```python
from build123d import *

# Parameters (mm, degrees)
SKETCH1_W           = 88
SKETCH1_H           = 92
BOSS_EXTRUDE1_DEPTH = 2
FILLET1_R           = 4
SKETCH3_W           = 28
SKETCH3_H           = 2
SKETCH3_W_2         = 9
BOSS_EXTRUDE3_DEPTH = 3
SKETCH4_W           = 2
SKETCH4_H           = 5
BOSS_EXTRUDE4_DEPTH = 6
FILLET2_R           = 2
BOSS_EXTRUDE5_DEPTH = 2
FILLET4_R           = 0.5


with BuildPart() as part:
    # Sketch1 → Boss-Extrude1 (new body)
    with BuildSketch(Plane.XY):
        with Locations((-29.854657196, 17.8829867)):
            Rectangle(SKETCH1_W, SKETCH1_H)
    extrude(amount=BOSS_EXTRUDE1_DEPTH)

    # Fillet1
    fillet1_edges = [part.edges().sort_by_distance(p)[0] for p in [
        (-73.854657196, 63.8829867, 1),
        (14.145342804, 63.8829867, 1),
    ]]
    fillet(fillet1_edges, radius=FILLET1_R)

    # Sketch3 → Boss-Extrude3 (add)
    with BuildSketch(Plane(origin=(0, 0, 0), x_dir=(-1, 0, 0), z_dir=(0, 0, -1))):
        with Locations((56.354657196, 62.8829867)):
            Rectangle(SKETCH3_W, SKETCH3_H)
        with Locations((29.854657196, 62.8829867)):
            Rectangle(SKETCH3_W_2, SKETCH3_H)
        with Locations((3.354657196, 62.8829867)):
            Rectangle(SKETCH3_W, SKETCH3_H)
    extrude(amount=BOSS_EXTRUDE3_DEPTH)

    # Sketch4 → Boss-Extrude4 (add)
    with BuildSketch(Plane(origin=(0, 0, 0), x_dir=(-1, 0, 0), z_dir=(0, 0, -1))):
        with Locations((-13.145342804, 21.3829867)):
            Rectangle(SKETCH4_W, SKETCH4_H)
    extrude(amount=BOSS_EXTRUDE4_DEPTH)

    # Fillet2
    fillet2_edges = [part.edges().sort_by_distance(p)[0] for p in [
        (14.145342804, -28.1170133, 1),
        (-73.854657196, -28.1170133, 1),
    ]]
    fillet(fillet2_edges, radius=FILLET2_R)

    # Sketch5 → Boss-Extrude5 (add)
    with BuildSketch(Plane(origin=(0, 0, 0), x_dir=(-1, 0, 0), z_dir=(0, 0, -1))):
        Polygon((71.854657196, -26.1170133), (68.854657196, -26.1170133), (-12.145342804, -26.1170133), (-12.145342804, -23.1170133), (-12.145342804, 54.889958553), (-9.145342804, 54.889958553), (-9.145342804, -23.1170133), (68.854657196, -23.1170133), (68.854657196, 54.749214955), (71.854657196, 54.749214955), align=None)
    extrude(amount=BOSS_EXTRUDE5_DEPTH)

    # Fillet4
    fillet4_edges = [part.edges().sort_by_distance(p)[0] for p in [
        (-71.854657196, 14.316100828, -2),
        (12.145342804, 39.386472626, -2),
        (12.145342804, -3.6170133, -2),
        (-29.854657196, -26.1170133, -2),
    ]]
    fillet(fillet4_edges, radius=FILLET4_R)


solid = part.part
```
Build history of the part. All positions in model axes, mm. A direction names the side the tool comes from. Round coordinates to 2 decimals unless told otherwise and drop trailing zeros. Write each loop counter-clockwise with the first axis right and the second up, starting at its lowest first coordinate (ties: lowest second). Pieces come first, ordered by that corner, then holes. Notation, with made-up numbers: (-6.5, -5) - (23.5, -5) arc R25 cw to (23.5, 21) - close; hole circle Ø7 at (-17.5, 42). An arc over 180 degrees is marked (long way). Write each question's results on one line, items separated by ' | '. Start each with the question number.
Item 1: Which spindle directions (+Z, -Z, +X, -X, +Y, -Y) get a long thin tool onto all of the face, cutting with end or side? Do faces 1 (the face through (10.645, 63, -1)), 2 (the face through (-30, 61.883, -1)), 3 (the face through (-68.855, 15, -1)), 4 (the face through (-34.355, 63, -1)). Say none if no direction does.
Item 2: Saw through at C-C (z = -4.5). Write the cut outline in (x, y).
Item 3: Saw through at B-B (y = -5). Write the cut outline in (x, z), and give its area (3 significant figures).
Item 4: Saw through at A-A (x = -60.5). Write the cut outline in (y, z), and give its area (3 significant figures).
Item 5: Drop flat-ended pins along their axis: P1, Ø2, axis at x = -70.5, z = -0.5, coming from the +Y side; P2, Ø1.5, axis at x = -28.5, z = -2, coming from the -Y side; P3, Ø0.6, axis at y = 62.5, z = -2, coming from the -X side; P4, Ø12, axis at x = -53, y = 15.5, coming from the -Z side. Give the stop position or say it passes through.
Item 6: Wall check: L1, parallel to Y at x = -47, z = -1; L2, parallel to X at y = 46.5, z = -1.5; L3, parallel to Z at x = -2, y = 24.5. Give the ranges that are in metal, low to high. Write a range as [from, to].
Item 7: Mould opens along X. For faces 5 (the face through (-29, -23.117, -1)), 6 (the face through (12.145, 21, -4)), 7 (the face through (-30, 63, -3)) say: pulls with the +X half, pulls with the -X half, needs draft (parallel to the pull), parting line crosses it, or undercut.
Results are:
1) face 1: -Z, +X, +Y | face 2: -Z, +X, -X | face 3: -Z | face 4: -Z, +Y
2) outline: (12.15, 18.88) - (14.15, 18.88) - (14.15, 23.88) - (12.15, 23.88) - close
3) outline: (-73.85, 0) - (-71.85, 0) - (-71.85, -1.5) arc R0.5 ccw to (-71.35, -2) - (-68.85, -2) - (-68.85, 0) - (9.15, 0) - (9.15, -2) - (11.65, -2) arc R0.5 ccw to (12.15, -1.5) - (12.15, 0) - (14.15, 0) - (14.15, 2) - (-73.85, 2) - close | area: 188 mm²
4) outline: (-28.12, 0) - (-26.12, 0) - (-26.12, -1.5) arc R0.5 ccw to (-25.62, -2) - (-23.12, -2) - (-23.12, 0) - (61.88, 0) - (61.88, -3) - (63.88, -3) - (63.88, 2) - (-28.12, 2) - close | area: 196 mm²
5) P1: stops at y = 63.88 | P2: stops at y = -26.12 | P3: stops at x = -70.35 | P4: stops at z = 0
6) L1: y = [-26.12, -23.12], [61.88, 63.88] | L2: x = [-71.85, -68.85], [9.15, 12.15] | L3: z = [0, 2]
7) face 5: undercut | face 6: pulls with the -X half | face 7: needs draft
